from build123d import *

# Parameters (mm, degrees)
F1_DEPTH = 38.1
F2_W     = 19.05
F2_H     = 107.95
F3_DEPTH = 152.4
F4_SIZE  = 31.75
F5_R     = 3.937
F6_DEPTH = 25.4


with BuildPart() as f1:
    # F0 (on Front) → F1 (new body)
    with BuildSketch(Plane.XZ):
        Polygon((0, 0), (9.30349, 0), (171.45, 0), (171.45, 19.05), (19.05, 19.05), (19.05, 127), (0, 127), align=None)
    extrude(amount=F1_DEPTH)

    # F2 (on face) → F3 (join, through all)
    with BuildSketch(Plane.YZ.offset(19.05)):
        with Locations((-9.525, 73.025)):
            Rectangle(F2_W, F2_H)
    extrude(amount=F3_DEPTH)

    # F4
    f4_edges = [f1.edges().sort_by_distance(p)[0] for p in [
        (171.45, -9.525, 127),
    ]]
    chamfer(f4_edges, length=F4_SIZE)

    # F5 (on face) → F6 (join)
    with BuildSketch(Plane.XZ.offset(19.05)):
        with Locations((50.8, 95.25)):
            Circle(F5_R)
        with Locations((127, 95.25)):
            Circle(F5_R)
        with Locations((127, 46.99)):
            Circle(F5_R)
        with Locations((50.8, 46.99)):
            Circle(F5_R)
    extrude(amount=F6_DEPTH)


solid = f1.part
Source: CAD feature listing. Evaluate the final solid. Frame: model axes, mm. A direction names the side the tool comes from. Round coordinates to 2 decimals unless told otherwise and drop trailing zeros. Loops run counter-clockwise (first coordinate to the right, second up) from the corner with the lowest first, then second, coordinate; pieces in that order, holes last. Notation, with made-up numbers: M 66,10 L 92,10 A19 cw 92,38 Z; hole C 48.5,1 d9. An arc over 180 degrees is marked long. Return JSON: item names as keys, results as strings. Group by question number.
1. Material intervals for line 1 along X through (y, z) = (-22.5, 43.5); line 2 along Y through (x, z) = (81, 7.5); line 3 along X through (y, z) = (-26, 48.5), sorted ascending. Write a range as from..to.
2. Section query D-D on z = 25. Output: boundary loops of the cut face in (x, y), and give its area (3 significant figures).
3. Pin query (flat end, axial travel): pin 1 (21 mm diameter, centred on y = -33, z = 57, fed in from +X); pin 2 (6 mm diameter, centred on y = -28.5, z = 71, fed in from +X); pin 3 (12 mm diameter, centred on x = 22, z = 15.5, fed in from -Y). Return the tip coordinate at first contact, or that it passes through.
4. Section query C-C on y = -4.5. Output: boundary loops of the cut face in (x, z).
5. Section query A-A on x = 50.8. Output: boundary loops of the cut face in (y, z).
6. Mould query, pull axis X, two halves, no side actions, for faces 1 (the face through (128.82, -31.57, 91.76)), 2 (the face through (85, -19, 0)), 3 (the face through (155.4, -9.7, 111.3)). Classes: released by +X, released by -X, zero draft, split by the parting line, or undercut.
7. Section query B-B on z = 46.99. Output: boundary loops of the cut face in (x, y).
8. Reachability of faces 4 (the face through (69, -11, 127)), 5 (the face through (19.05, -28, 72)), 6 (the face through (130.637, -31.572, 45.482)) from +Z, -Z, +X, -X, +Y, -Y: full face, straight path, thin tool, end or side. Return the list, or none.
Checks:
{
 "1": {"line 1": "x = 0..19.05, 48.98..52.62, 125.18..128.82", "line 2": "y = -38.1..0", "line 3": "x = 0..19.05, 47.16..54.44, 123.36..130.64"},
 "2": {"outline": "M 0,-38.1 L 19.05,-38.1 L 19.05,-19.05 L 171.45,-19.05 L 171.45,0 L 0,0 Z", "area": "3,630 mm²"},
 "3": {"pin 1": "stops at x = 130.94", "pin 2": "stops at x = 19.05", "pin 3": "stops at y = -38.1"},
 "4": {"outline": "M 0,0 L 171.45,0 L 171.45,95.25 L 139.7,127 L 0,127 Z"},
 "5": {"outline": "M -44.45,43.05 L -19.05,43.05 L -19.05,19.05 L -38.1,19.05 L -38.1,0 L 0,0 L 0,127 L -19.05,127 L -19.05,99.19 L -44.45,99.19 L -44.45,91.31 L -19.05,91.31 L -19.05,50.93 L -44.45,50.93 Z"},
 "6": {"face 1": "undercut", "face 2": "zero draft", "face 3": "released by +X"},
 "7": {"outline": "M 0,-38.1 L 19.05,-38.1 L 19.05,-19.05 L 46.86,-19.05 L 46.86,-44.45 L 54.74,-44.45 L 54.74,-19.05 L 123.06,-19.05 L 123.06,-44.45 L 130.94,-44.45 L 130.94,-19.05 L 171.45,-19.05 L 171.45,0 L 0,0 Z"},
 "8": {"face 4": "+Z, +X, -X, +Y, -Y", "face 5": "+Z, -Y", "face 6": "-Y"}
}
